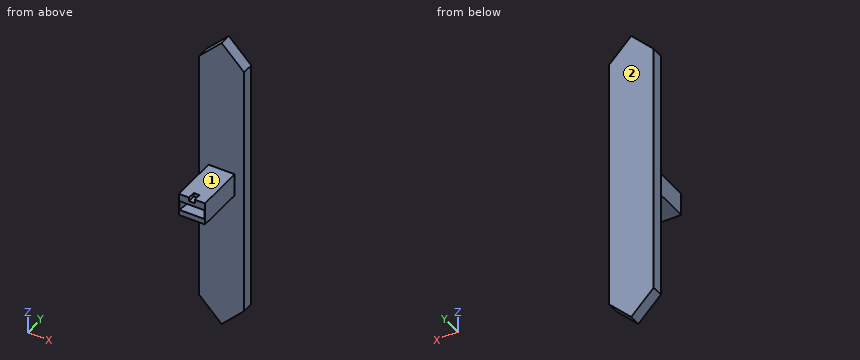
```python
from build123d import *

# Parameters (mm, degrees)
BOSS_EXTRUDE1_DEPTH = 3.125
SKETCH2_W           = 7
SKETCH2_H           = 4
BOSS_EXTRUDE2_DEPTH = 13
CUT_EXTRUDE1_DEPTH  = 2.5
SKETCH4_W           = 7
SKETCH4_H           = 13
BOSS_EXTRUDE3_DEPTH = 2
SKETCH5_W           = 1.55719089
SKETCH5_H           = 4.099138032
CUT_EXTRUDE2_DEPTH  = 1


with BuildPart() as part:
    # Sketch1 → Boss-Extrude1 (new body)
    with BuildSketch(Plane(origin=(0, 0, 0), x_dir=(1, 0, 0), z_dir=(0, 1, 0))):
        Polygon((0, 0), (6, -6), (6, -74), (0, -80), (-6, -74), (-6, -6), align=None)
    extrude(amount=BOSS_EXTRUDE1_DEPTH)

    # Sketch2 → Boss-Extrude2 (add)
    with BuildSketch(Plane.XZ):
        with Locations((0, 40)):
            Rectangle(SKETCH2_W, SKETCH2_H)
    extrude(amount=BOSS_EXTRUDE2_DEPTH)

    # Sketch3 → Cut-Extrude1 (cut)
    with BuildSketch(Plane.XY.offset(42)):
        with BuildLine():
            Line((3.5, -14.64), (-3.5, -14.64))
            Line((-3.5, -14.64), (-2.25, -2.8))
            ThreePointArc((-2.25, -2.8), (0, -0.55), (2.25, -2.8))
            Line((2.25, -2.8), (3.5, -14.64))
        make_face()
    extrude(amount=-CUT_EXTRUDE1_DEPTH, mode=Mode.SUBTRACT)

    # Sketch4 → Boss-Extrude3 (add)
    with BuildSketch(Plane.XY.offset(42)):
        with Locations((0, -6.5)):
            Rectangle(SKETCH4_W, SKETCH4_H)
    extrude(amount=BOSS_EXTRUDE3_DEPTH)

    # Sketch5 → Cut-Extrude2 (cut)
    with BuildSketch(Plane.XY.offset(44)):
        with Locations((0, -13)):
            Rectangle(SKETCH5_W, SKETCH5_H)
    extrude(amount=-CUT_EXTRUDE2_DEPTH, mode=Mode.SUBTRACT)


solid = part.part
```
Geometry check sheet. Reference: the model listing, model coordinates, mm. Face numbers are marked on the shaded views. A direction names the side the tool comes from. Give positions to 0.01 mm unless a question says otherwise; leave off trailing zeros. Write each loop counter-clockwise with the first axis right and the second up, starting at its lowest first coordinate (ties: lowest second). Pieces come first, ordered by that corner, then holes.
1) Gauge pin test, flat ends, axial feed: pin 1 (6.5 mm diameter, centred on y = -8.5, z = 41.5, fed in from -X); pin 2 (1.1 mm diameter, centred on y = -11.5, z = 43.5, fed in from +X); pin 3 (4 mm diameter, centred on x = 3.5, y = -6, fed in from -Z). Record the tip position at first contact, or that the pin passes through.
2) Material ranges on L1, parallel to Z at x = 1.5, y = -4.75; L2, parallel to Y at x = 2, z = 67 (3 decimals); L3, parallel to Z at x = -0.5, y = 2.25, recorded low to high.
3) Section check B-B, the plane z = 61. Record the boundary of the cut face in (x, y) (3 decimals), and give its area (3 significant figures).
4) Section check C-C, the plane y = -4.5. Record the boundary of the cut face in (x, z), and give its area (3 significant figures).
5) Section check A-A, the plane y = -9.25. Record the boundary of the cut face in (x, z).
6) Section check D-D, the plane z = 75.5. Record the boundary of the cut face in (x, y) (3 decimals), and give its area (3 significant figures).
7) Access from +Z, -Z, +X, -X, +Y, -Y to the whole of each face (thin tool, end or side, straight path). Record for the marked faces 1 and 2.
Computed:
1. pin 1: stops at x = -3.5
1. pin 2: stops at x = 3.5
1. pin 3: stops at z = 38
2. L1: z = 38 to 39.5, 42 to 44
2. L2: y = 0 to 3.125
2. L3: z = 0.5 to 79.5
3. outline: (-6, 0) - (6, 0) - (6, 3.125) - (-6, 3.125) - close
3. area: 37.5 mm2
4. outline: (-3.5, 38) - (3.5, 38) - (3.5, 44) - (-3.5, 44) - close; hole (-2.43, 39.5) - (2.43, 39.5) - (2.43, 42) - (-2.43, 42) - close
4. area: 29.9 mm2
5. outline: (-3.5, 38) - (3.5, 38) - (3.5, 44) - (-3.5, 44) - close; hole (-2.93, 39.5) - (2.93, 39.5) - (2.93, 42) - (-2.93, 42) - close
6. outline: (-4.5, 0) - (4.5, 0) - (4.5, 3.125) - (-4.5, 3.125) - close
6. area: 28.1 mm2
7. face 1: +Z, +X, -X, -Y
7. face 2: +Z, -Z, +X, -X, +Y
